Study the drawing (mm; zero at the part's minimum x, y, z) and answer. Coordinates: 2 decimals unless noted, no trailing zeros. Write each loop counter-clockwise with the first axis right and the second up, starting at its lowest first coordinate (ties: lowest second). Pieces come first, ordered by that corner, then holes. Notation, with made-up numbers: M 45,57 L 51,57 A10 ccw 51,71 Z; hole C 12.25,-10 d3. An arc over 180 degrees is marked long. Answer as CSV lines item,"result". Start each with the question number.
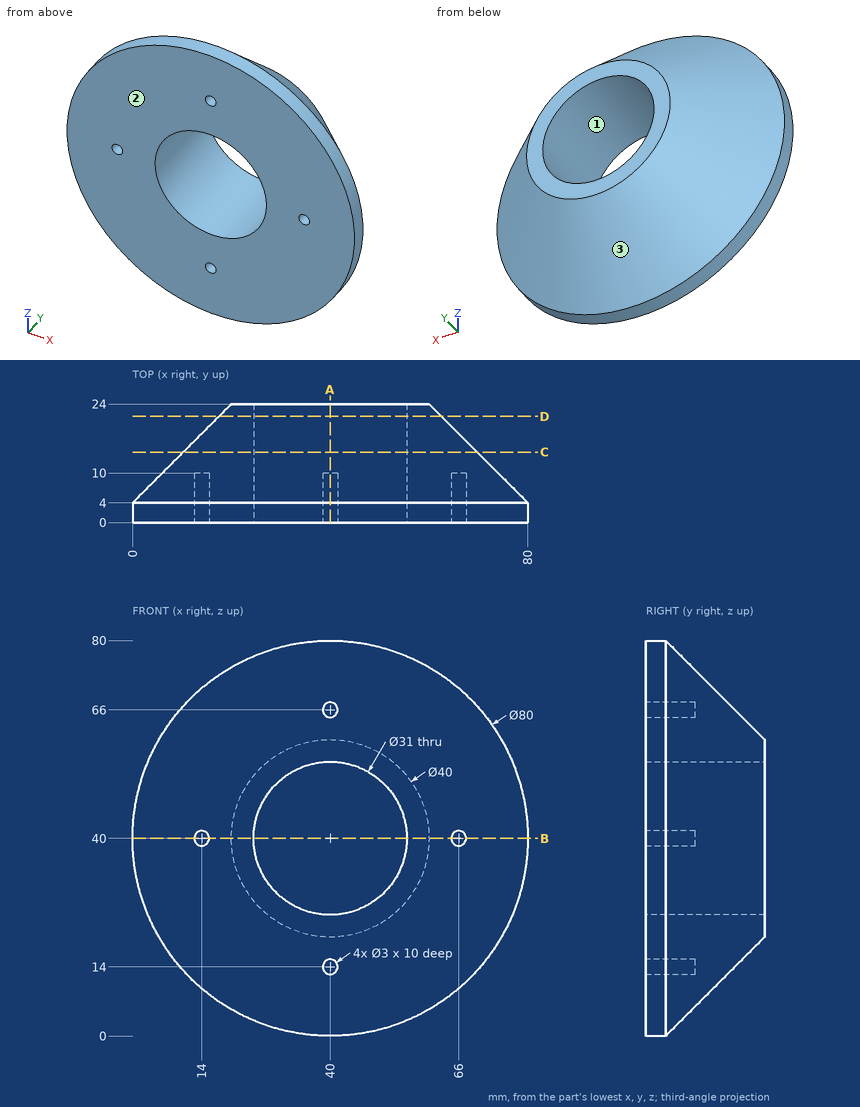
1) For a pull along X with two mould halves and no side action, classify the marked faces 1, 2 and 3 as +X half, -X half, draft (parallel to the pull), parting line (faces both ways), or undercut.
2) The part is cut by section C-C (y = 14.25). Determine the outline of the cut face in (x, z).
3) Each of these flat-tipped pins is pushed along its axis until it touches: P1, Ø3, axis at y = 12, z = 32.5, coming from the +X side; P2, Ø3.5, axis at x = 13.5, z = 40.5, coming from the -Y side; P3, Ø0.9, axis at x = 40, z = 66.5, coming from the -Y side; P4, Ø1, axis at y = 18.5, z = 44.5, coming from the +X side (3 decimals). Where does it stop, or does it pass through?
4) The part is cut by section A-A (x = 40). Determine the outline of the cut face in (y, z).
5) Find the intervals of material crossed by line 1 (X direction, y = 4, z = 40); line 2 (X direction, y = 7.75, z = 40); line 3 (Z direction, x = 37.5, y = 7.5), in increasing order. Write a range as from..to.
6) The part is cut by section D-D (y = 21.5). Determine the outline of the cut face in (x, z), then the cut area to 3 significant figures.
7) The part is cut by section B-B (z = 40). Determine the outline of the cut face in (x, y).
Completed:
1,face 1,"undercut"
1,face 2,"draft"
1,face 3,"parting line"
2,outline,"C 40,40 d59.5; hole C 40,40 d31"
3,P1,"x = 72.69"
3,P2,"y = 0"
3,P3,"y = 10"
3,P4,"x = 65.615"
4,outline,"M 0,0 L 4,0 L 24,20 L 24,24.5 L 0,24.5 L 0,15.5 L 10,15.5 L 10,12.5 L 0,12.5 Z; M 0,55.5 L 24,55.5 L 24,60 L 4,80 L 0,80 L 0,67.5 L 10,67.5 L 10,64.5 L 0,64.5 Z"
5,line 1,"0..12.5, 15.5..24.5, 55.5..64.5, 67.5..80"
5,line 2,"3.75..12.5, 15.5..24.5, 55.5..64.5, 67.5..76.25"
5,line 3,"3.59..24.7, 55.3..76.41"
6,outline,"C 40,40 d45; hole C 40,40 d31"
6,area,"836 mm²"
7,outline,"M 0,0 L 12.5,0 L 12.5,10 L 15.5,10 L 15.5,0 L 24.5,0 L 24.5,24 L 20,24 L 0,4 Z; M 55.5,0 L 64.5,0 L 64.5,10 L 67.5,10 L 67.5,0 L 80,0 L 80,4 L 60,24 L 55.5,24 Z"
